from build123d import *

# Parameters (mm, degrees)
SKETCH1_W            = 28.6
SKETCH1_H            = 10.6
SKETCH1_W_2          = 25.6
SKETCH1_H_2          = 7.6
BOSS_EXTRUDE1_DEPTH  = 55
SKETCH2_W            = 36.6
SKETCH2_H            = 18.6
SKETCH2_W_2          = 25.6
SKETCH2_H_2          = 7.6
BOSS_EXTRUDE3_DEPTH  = 3
FILLET2_R            = 2
FILLET1_R            = 2
FILLET2_OF_MIRROR2_R = 2
FILLET3_R            = 2


with BuildPart() as part:
    # Sketch1 → Boss-Extrude1 (new body)
    with BuildSketch(Plane.XY):
        Rectangle(SKETCH1_W, SKETCH1_H)
        Rectangle(SKETCH1_W_2, SKETCH1_H_2, mode=Mode.SUBTRACT)
    extrude(amount=BOSS_EXTRUDE1_DEPTH)

    # Sketch2 → Boss-Extrude3 (add)
    with BuildSketch(Plane.XY.offset(55)):
        Rectangle(SKETCH2_W, SKETCH2_H)
        Rectangle(SKETCH2_W_2, SKETCH2_H_2, mode=Mode.SUBTRACT)
    boss_extrude3 = extrude(amount=BOSS_EXTRUDE3_DEPTH)

    # Fillet2
    fillet2_edges = [part.edges().sort_by_distance(p)[0] for p in [
        (18.3, -9.3, 56.5),
        (18.3, 9.3, 56.5),
        (-18.3, 9.3, 56.5),
        (-18.3, -9.3, 56.5),
    ]]
    fillet(fillet2_edges, radius=FILLET2_R)

    # Fillet1
    fillet1_edges = [part.edges().sort_by_distance(p)[0] for p in [
        (14.3, -5.3, 27.5),
        (-14.3, -5.3, 27.5),
        (-14.3, 5.3, 27.5),
        (14.3, 5.3, 27.5),
    ]]
    fillet(fillet1_edges, radius=FILLET1_R)

    # Mirror2: Boss-Extrude3 across plane
    add(boss_extrude3.mirror(Plane(origin=(0, 0, 27.5), x_dir=(1, 0, 0), z_dir=(0, 0, -1))))

    # Fillet2 of Mirror2
    fillet2_of_mirror2_edges = [part.edges().sort_by_distance(p)[0] for p in [
        (18.3, -9.3, -1.5),
        (18.3, 9.3, -1.5),
        (-18.3, 9.3, -1.5),
        (-18.3, -9.3, -1.5),
    ]]
    fillet(fillet2_of_mirror2_edges, radius=FILLET2_OF_MIRROR2_R)

    # Fillet3
    fillet3_edges = [part.edges().sort_by_distance(p)[0] for p in [
        (12.8, -3.8, 27.5),
        (12.8, 3.8, 27.5),
        (-12.8, 3.8, 27.5),
        (-12.8, -3.8, 27.5),
    ]]
    fillet(fillet3_edges, radius=FILLET3_R)


solid = part.part
Verification items for the finished model (mm, model axes). A direction names the side the tool comes from. Give positions to 0.01 mm unless a question says otherwise; leave off trailing zeros. Write each loop counter-clockwise with the first axis right and the second up, starting at its lowest first coordinate (ties: lowest second). Pieces come first, ordered by that corner, then holes. Notation, with made-up numbers: (-27.75, 19) - (-6.75, 19) arc R21 ccw to (-6.75, 27) - close; hole circle Ø7 at (15, -8). An arc over 180 degrees is marked (long way). Answer as CSV lines item,"result". Start each with the question number.
1. Thickness scan on line 1 (Y direction, x = -7, z = 21); line 2 (X direction, y = 1, z = 39.5); line 3 (Z direction, x = 15, y = 1). Record the ranges inside material, lowest first.
2. Sectioned sample at C-C (x = -7.5). Record the boundary of the cut face in (y, z), then the cut area to 3 significant figures.
3. Draft check along Y on faces 4 (the face through (12.23, 3.2, 27.07)), 5 (the face through (-17.73, -8.7, 56.52)), 6 (the face through (0, 4, -3)). Enter one of: pulls with the +Y half, pulls with the -Y half, needs draft (parallel to the pull), parting line crosses it, or undercut.
4. Sectioned sample at A-A (y = -6). Record the boundary of the cut face in (x, z), then the cut area to 3 significant figures.
5. Set-up check for faces 1 (the face through (13.73, 4.7, 27.88)), 2 (the face through (-12.8, 0, 28)), 3 (the face through (0, 5.3, 27)): record each of +Z, -Z, +X, -X, +Y, -Y from which the full face is reachable in a straight line by a thin tool's end or side.
6. Sectioned sample at B-B (z = 49.5). Record the boundary of the cut face in (x, y).
7. Sectioned sample at D-D (y = -0.75). Record the boundary of the cut face in (x, z).
8. Depth check by flat-ended pin: pin 1 (19.5 mm diameter, centred on x = 2, z = 17.5, fed in from -Y); pin 2 (3.5 mm diameter, centred on y = -0.5, z = 31.5, fed in from +X); pin 3 (17.5 mm diameter, centred on x = 0.5, z = 34, fed in from +Y); pin 4 (1 mm diameter, centred on x = 4.5, y = -3, fed in from +Z). Enter the tip coordinate at first touch or a pass-through.
Derived:
1,line 1,"-5.3 to -3.8, 3.8 to 5.3"
1,line 2,"-14.3 to -12.8, 12.8 to 14.3"
1,line 3,"-3 to 0, 55 to 58"
2,outline,"(-9.3, -3) - (-3.8, -3) - (-3.8, 58) - (-9.3, 58) - (-9.3, 55) - (-5.3, 55) - (-5.3, 0) - (-9.3, 0) - close; (3.8, -3) - (9.3, -3) - (9.3, 0) - (5.3, 0) - (5.3, 55) - (9.3, 55) - (9.3, 58) - (3.8, 58) - close"
2,area,"231 mm²"
3,face 4,"undercut"
3,face 5,"pulls with the -Y half"
3,face 6,"needs draft"
4,outline,"(-18.3, -3) - (18.3, -3) - (18.3, 0) - (-18.3, 0) - close; (-18.3, 55) - (18.3, 55) - (18.3, 58) - (-18.3, 58) - close"
4,area,"220 mm²"
5,face 1,"+X, +Y"
5,face 2,"+Z, -Z"
5,face 3,"+X, -X, +Y"
6,outline,"(-14.3, -3.3) arc R2 ccw to (-12.3, -5.3) - (12.3, -5.3) arc R2 ccw to (14.3, -3.3) - (14.3, 3.3) arc R2 ccw to (12.3, 5.3) - (-12.3, 5.3) arc R2 ccw to (-14.3, 3.3) - close; hole (-12.8, -1.8) arc R2 ccw to (-10.8, -3.8) - (10.8, -3.8) arc R2 ccw to (12.8, -1.8) - (12.8, 1.8) arc R2 ccw to (10.8, 3.8) - (-10.8, 3.8) arc R2 ccw to (-12.8, 1.8) - close"
7,outline,"(-18.3, -3) - (-12.8, -3) - (-12.8, 58) - (-18.3, 58) - (-18.3, 55) - (-14.3, 55) - (-14.3, 0) - (-18.3, 0) - close; (12.8, -3) - (18.3, -3) - (18.3, 0) - (14.3, 0) - (14.3, 55) - (18.3, 55) - (18.3, 58) - (12.8, 58) - close"
8,pin 1,"y = -5.3"
8,pin 2,"x = 14.3"
8,pin 3,"y = 5.3"
8,pin 4,"through"
